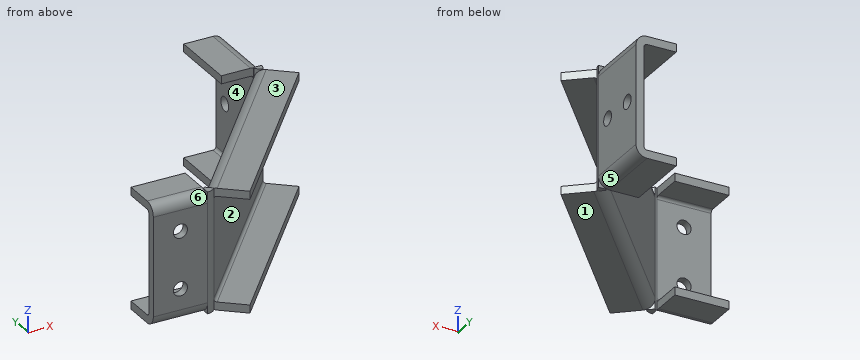
from build123d import *

# Parameters (mm, degrees)
BASE_FLANGE1_DEPTH             = 30
EDGE_FLANGE1_STRIP_W           = 9.4732
EDGE_FLANGE1_STRIP_H           = 2
EDGE_FLANGE1_STRIP_CUT_DEPTH   = 16.803293835
EDGE_FLANGE1_STRIP_2_W         = 9.4732
EDGE_FLANGE1_STRIP_2_H         = 2
EDGE_FLANGE1_STRIP_CUT_2_DEPTH = 13.476690823
EDGE_FLANGE1_STRIP_3_W         = 9.4732
EDGE_FLANGE1_STRIP_3_H         = 2
EDGE_FLANGE1_STRIP_CUT_3_DEPTH = 16.803293835
EDGE_FLANGE1_STRIP_4_W         = 9.4732
EDGE_FLANGE1_STRIP_4_H         = 2
EDGE_FLANGE1_STRIP_CUT_4_DEPTH = 13.476690823
EDGE_FLANGE1_DEPTH             = 16.803293835
EDGE_FLANGE1_BEND_DEPTH        = 13.476690823
EDGE_FLANGE1_BEND_2_DEPTH      = 16.803293835
EDGE_FLANGE1_BEND_3_DEPTH      = 13.476690823
EDGE_FLANGE2_STRIP_W           = 9.4732
EDGE_FLANGE2_STRIP_H           = 2
EDGE_FLANGE2_STRIP_CUT_DEPTH   = 55.838043997
EDGE_FLANGE2_STRIP_2_W         = 9.4732
EDGE_FLANGE2_STRIP_2_H         = 2
EDGE_FLANGE2_STRIP_CUT_2_DEPTH = 55.838043997
EDGE_FLANGE2_DEPTH             = 55.838043997
EDGE_FLANGE2_BEND_DEPTH        = 55.838043997
SKETCH32_R                     = 1.75
CUT_EXTRUDE1_DEPTH             = 10
SKETCH33_R                     = 1.75
CUT_EXTRUDE2_DEPTH             = 10


# Sheet-metal steps are written as plain solids
with BuildPart() as part:
    # Sketch1 → Base-Flange1 (new body)
    with BuildSketch(Plane.XY):
        with BuildLine():
            Line((0, 0), (13.476690823, 0))
            ThreePointArc((13.476690823, 0), (13.787790598, 0.068920069), (14.040674196, 0.262783248))
            Line((14.040674196, 0.262783248), (49.95840521, 43.015604865))
            ThreePointArc((49.95840521, 43.015604865), (50.086523604, 43.237281371), (50.131021837, 43.489421617))
            Line((50.131021837, 43.489421617), (50.131021837, 60.292715453))
            Line((50.131021837, 60.292715453), (52.131021837, 60.292715453))
            Line((52.131021837, 60.292715453), (52.131021837, 43.489421617))
            ThreePointArc((52.131021837, 43.489421617), (51.965702989, 42.552675762), (51.489720369, 41.729108117))
            Line((51.489720369, 41.729108117), (15.571989355, -1.023713501))
            ThreePointArc((15.571989355, -1.023713501), (14.632481815, -1.743949686), (13.476690823, -2))
            Line((13.476690823, -2), (0, -2))
            Line((0, -2), (0, 0))
        make_face()
    extrude(amount=BASE_FLANGE1_DEPTH)

    # Edge-Flange1 strip (across the edge) → Edge-Flange1 strip cut (cut)
    with BuildSketch(Plane(origin=(50.131021837, 43.489421617, 30), x_dir=(0, 0, -1), z_dir=(0, 1, 0))):
        with Locations((-2, -1)):
            Rectangle(EDGE_FLANGE1_STRIP_W, EDGE_FLANGE1_STRIP_H)
    extrude(amount=EDGE_FLANGE1_STRIP_CUT_DEPTH, mode=Mode.SUBTRACT)

    # Edge-Flange1 strip 2 (across the edge) → Edge-Flange1 strip cut 2 (cut)
    with BuildSketch(Plane(origin=(0, 0, 30), x_dir=(0, 0, -1), z_dir=(1, 0, 0))):
        with Locations((-2, -1)):
            Rectangle(EDGE_FLANGE1_STRIP_2_W, EDGE_FLANGE1_STRIP_2_H)
    extrude(amount=EDGE_FLANGE1_STRIP_CUT_2_DEPTH, mode=Mode.SUBTRACT)

    # Edge-Flange1 strip 3 (across the edge) → Edge-Flange1 strip cut 3 (cut)
    with BuildSketch(Plane(origin=(50.131021837, 60.292715453, 0), x_dir=(0, 0, 1), z_dir=(0, -1, 0))):
        with Locations((-2, -1)):
            Rectangle(EDGE_FLANGE1_STRIP_3_W, EDGE_FLANGE1_STRIP_3_H)
    extrude(amount=EDGE_FLANGE1_STRIP_CUT_3_DEPTH, mode=Mode.SUBTRACT)

    # Edge-Flange1 strip 4 (across the edge) → Edge-Flange1 strip cut 4 (cut)
    with BuildSketch(Plane.ZY.offset(-13.476690823)):
        with Locations((-2, -1)):
            Rectangle(EDGE_FLANGE1_STRIP_4_W, EDGE_FLANGE1_STRIP_4_H)
    extrude(amount=EDGE_FLANGE1_STRIP_CUT_4_DEPTH, mode=Mode.SUBTRACT)

    # Edge-Flange1 section (across the edge) → Edge-Flange1 (add)
    with BuildSketch(Plane(origin=(50.131021837, 43.489421617, 30), x_dir=(0, 0, -1), z_dir=(0, 1, 0))):
        with BuildLine():
            Line((0, 0.7366), (0, 8))
            Line((0, 8), (2, 8))
            Line((2, 8), (2, 0.7366))
            ThreePointArc((2, 0.7366), (2.215745145, 0.215745145), (2.7366, 0))
            Line((2.7366, 0), (2.7366, -2))
            ThreePointArc((2.7366, -2), (0.801531583, -1.198468417), (0, 0.7366))
        make_face()
    extrude(amount=EDGE_FLANGE1_DEPTH)

    # Edge-Flange1 section 2 (across the edge) → Edge-Flange1 bend (add)
    with BuildSketch(Plane(origin=(0, 0, 30), x_dir=(0, 0, -1), z_dir=(1, 0, 0))):
        with BuildLine():
            Line((0, 0.7366), (0, 8))
            Line((0, 8), (2, 8))
            Line((2, 8), (2, 0.7366))
            ThreePointArc((2, 0.7366), (2.215745145, 0.215745145), (2.7366, 0))
            Line((2.7366, 0), (2.7366, -2))
            ThreePointArc((2.7366, -2), (0.801531583, -1.198468417), (0, 0.7366))
        make_face()
    extrude(amount=EDGE_FLANGE1_BEND_DEPTH)

    # Edge-Flange1 section 3 (across the edge) → Edge-Flange1 bend 2 (add)
    with BuildSketch(Plane(origin=(50.131021837, 60.292715453, 0), x_dir=(0, 0, 1), z_dir=(0, -1, 0))):
        with BuildLine():
            Line((0, 0.7366), (0, 8))
            Line((0, 8), (2, 8))
            Line((2, 8), (2, 0.7366))
            ThreePointArc((2, 0.7366), (2.215745145, 0.215745145), (2.7366, 0))
            Line((2.7366, 0), (2.7366, -2))
            ThreePointArc((2.7366, -2), (0.801531583, -1.198468417), (0, 0.7366))
        make_face()
    extrude(amount=EDGE_FLANGE1_BEND_2_DEPTH)

    # Edge-Flange1 section 4 (across the edge) → Edge-Flange1 bend 3 (add)
    with BuildSketch(Plane.ZY.offset(-13.476690823)):
        with BuildLine():
            Line((0, 0.7366), (0, 8))
            Line((0, 8), (2, 8))
            Line((2, 8), (2, 0.7366))
            ThreePointArc((2, 0.7366), (2.215745145, 0.215745145), (2.7366, 0))
            Line((2.7366, 0), (2.7366, -2))
            ThreePointArc((2.7366, -2), (0.801531583, -1.198468417), (0, 0.7366))
        make_face()
    extrude(amount=EDGE_FLANGE1_BEND_3_DEPTH)

    # Edge-Flange2 strip (across the edge) → Edge-Flange2 strip cut (cut)
    with BuildSketch(Plane(origin=(51.489720369, 41.729108117, 30), x_dir=(0, 0, -1), z_dir=(-0.6432483740966664, -0.7656575796150621, 0))):
        with Locations((-2, -1)):
            Rectangle(EDGE_FLANGE2_STRIP_W, EDGE_FLANGE2_STRIP_H)
    extrude(amount=EDGE_FLANGE2_STRIP_CUT_DEPTH, mode=Mode.SUBTRACT)

    # Edge-Flange2 strip 2 (across the edge) → Edge-Flange2 strip cut 2 (cut)
    with BuildSketch(Plane(origin=(15.571989355, -1.023713501, 0), x_dir=(0, 0, 1), z_dir=(0.6432483740966664, 0.7656575796150621, 0))):
        with Locations((-2, -1)):
            Rectangle(EDGE_FLANGE2_STRIP_2_W, EDGE_FLANGE2_STRIP_2_H)
    extrude(amount=EDGE_FLANGE2_STRIP_CUT_2_DEPTH, mode=Mode.SUBTRACT)

    # Edge-Flange2 section (across the edge) → Edge-Flange2 (add)
    with BuildSketch(Plane(origin=(51.489720369, 41.729108117, 30), x_dir=(0, 0, -1), z_dir=(-0.6432483740966664, -0.7656575796150621, 0))):
        with BuildLine():
            Line((0, 0.7366), (0, 8))
            Line((0, 8), (2, 8))
            Line((2, 8), (2, 0.7366))
            ThreePointArc((2, 0.7366), (2.215745145, 0.215745145), (2.7366, 0))
            Line((2.7366, 0), (2.7366, -2))
            ThreePointArc((2.7366, -2), (0.801531583, -1.198468417), (0, 0.7366))
        make_face()
    extrude(amount=EDGE_FLANGE2_DEPTH)

    # Edge-Flange2 section 2 (across the edge) → Edge-Flange2 bend (add)
    with BuildSketch(Plane(origin=(15.571989355, -1.023713501, 0), x_dir=(0, 0, 1), z_dir=(0.6432483740966664, 0.7656575796150621, 0))):
        with BuildLine():
            Line((0, 0.7366), (0, 8))
            Line((0, 8), (2, 8))
            Line((2, 8), (2, 0.7366))
            ThreePointArc((2, 0.7366), (2.215745145, 0.215745145), (2.7366, 0))
            Line((2.7366, 0), (2.7366, -2))
            ThreePointArc((2.7366, -2), (0.801531583, -1.198468417), (0, 0.7366))
        make_face()
    extrude(amount=EDGE_FLANGE2_BEND_DEPTH)

    # Sketch32 → Cut-Extrude1 (cut)
    with BuildSketch(Plane(origin=(0, 0, 0), x_dir=(1, 0, 0), z_dir=(0, 1, 0))):
        with Locations(Location((6.738345411, -7.891027615, 0), (0, 0, 270))):
            Circle(SKETCH32_R)
        with Locations(Location((6.738345411, -22.108972385, 0), (0, 0, 270))):
            Circle(SKETCH32_R)
    extrude(amount=-CUT_EXTRUDE1_DEPTH, mode=Mode.SUBTRACT)

    # Sketch33 → Cut-Extrude2 (cut)
    with BuildSketch(Plane.ZY.offset(-50.131021837)):
        with Locations((15, 56.35303153)):
            Circle(SKETCH33_R)
        with Locations((15, 47.577872809)):
            Circle(SKETCH33_R)
    extrude(amount=-CUT_EXTRUDE2_DEPTH, mode=Mode.SUBTRACT)


solid = part.part
Could you check a few things on this model? Use its own coordinates, in mm. Face numbers are marked on the shaded views. A direction names the side the tool comes from. Coordinates: 2 decimals unless noted, no trailing zeros. Order: outer loops, then holes, each group sorted by start corner. A loop starts at its lowest first (then second) coordinate and runs counter-clockwise, first axis right, second up. Notation, with made-up numbers: (0.25, -22) -> (51.25, -22) arc R24 ccw to (51.25, -11) -> close; hole circle Ø1 at (79, 46). An arc over 180 degrees is marked (long way). One line per item, written item: value. Start each with the question number.
1) Which directions (+Z, -Z, +X, -X, +Y, -Y) give clear straight access to the entire face, cutting with the end or side of a thin tool? Please do the marked faces 4, 5 and 6.
2) Imagine slicing it at A-A on z = 15. List the corners of the cut face in (x, y) for me.
3) If I drill on L1, parallel to Z at x = 30, y = 14.5; L2, parallel to Y at x = 51.45, z = 15; L3, parallel to X at y = 47.5, z = 23, over which ranges is the centre line in solid material (lowest first)? Write a range as [from, to].
4) We'd pull the mould along Z, two halves only. Please class the marked faces 1, 2 and 3: +Z half, -Z half, draft (parallel to the pull), parting line (faces both ways), or undercut.
5) Imagine slicing it at B-B on x = 54. List the corners of the cut face in (y, z) for me, plus the area to 3 significant figures.
6) Imagine slicing it at C-C on z = 4.25. List the corners of the cut face in (x, y) for me, plus the area to 3 significant figures.
7) I'm going to push flat-ended pins straight in: pin 1 (2 mm diameter, centred on y = 22, z = 12, fed in from +X); pin 2 (1 mm diameter, centred on x = 19, z = 12, fed in from +Y); pin 3 (1.6 mm diameter, centred on y = 53, z = 28.5, fed in from -X). Where does each tip first touch, or does it pass through?
8) Imagine slicing it at D-D on x = 11.5. List the corners of the cut face in (y, z) for me, plus the area to 3 significant figures.
Answer list:
1. face 4: -X, +Y
1. face 5: -Z, +X, +Y
1. face 6: +Z, -X, -Y
2. outline: (0, -2) -> (13.48, -2) arc R2.74 ccw to (15.57, -1.02) -> (51.49, 41.73) arc R2.74 ccw to (52.13, 43.49) -> (52.13, 45.83) -> (50.13, 45.83) -> (50.13, 43.49) arc R0.74 cw to (49.96, 43.02) -> (14.04, 0.26) arc R0.74 cw to (13.48, 0) -> (0, 0) -> close; (50.13, 49.33) -> (52.13, 49.33) -> (52.13, 54.6) -> (50.13, 54.6) -> close; (50.13, 58.1) -> (52.13, 58.1) -> (52.13, 60.29) -> (50.13, 60.29) -> close
3. L1: z = [0, 2], [28, 30]
3. L2: y = [41.68, 45.83], [49.33, 54.6], [58.1, 60.29]
3. L3: x = [50.13, 52.13]
4. face 1: -Z half
4. face 2: undercut
4. face 3: +Z half
5. outline: (32.28, 0) -> (39.62, 0) -> (39.62, 2) -> (32.28, 2) -> close; (32.28, 28) -> (39.62, 28) -> (39.62, 30) -> (32.28, 30) -> close
5. area: 29.4 mm2
6. outline: (0, -2) -> (13.48, -2) arc R2.74 ccw to (15.57, -1.02) -> (51.49, 41.73) arc R2.74 ccw to (52.13, 43.49) -> (52.13, 60.29) -> (50.13, 60.29) -> (50.13, 43.49) arc R0.74 cw to (49.96, 43.02) -> (14.04, 0.26) arc R0.74 cw to (13.48, 0) -> (0, 0) -> close
6. area: 178 mm2
7. pin 1: stops at x = 35.75
7. pin 2: stops at y = 6.76
7. pin 3: stops at x = 42.13
8. outline: (-2, 2.74) arc R2.74 ccw to (0.74, 0) -> (8, 0) -> (8, 2) -> (0.74, 2) arc R0.74 cw to (0, 2.74) -> (0, 27.26) arc R0.74 cw to (0.74, 28) -> (8, 28) -> (8, 30) -> (0.74, 30) arc R2.74 ccw to (-2, 27.26) -> close
8. area: 89.0 mm2
